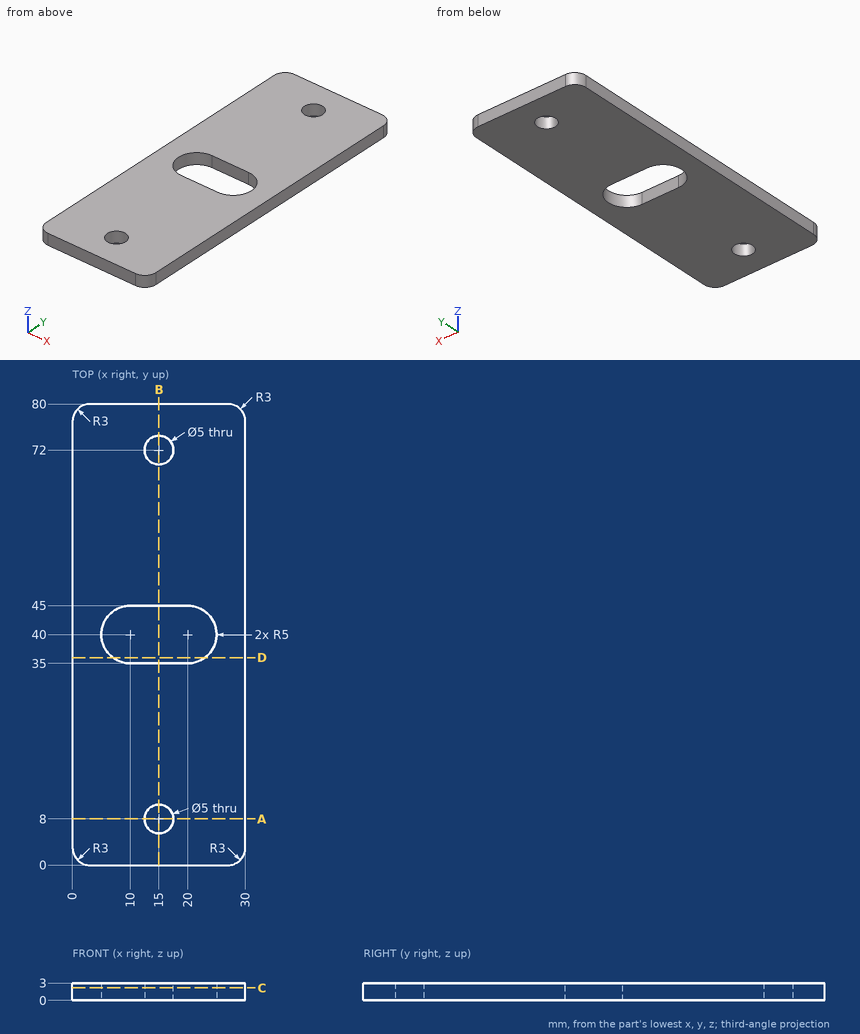
Could you check a few things on this drawing? It's one solid part, dimensions in mm from its lowest x, y, z. Coordinates: 2 decimals unless noted, no trailing zeros. Loops run counter-clockwise (first coordinate to the right, second up) from the corner with the lowest first, then second, coordinate; pieces in that order, holes last.
1. I need wall thicknesses on L1, parallel to Y at x = 15, z = 0.85; L2, parallel to X at y = 72, z = 2.15; L3, parallel to Y at x = 18, z = 2.2. Which ranges of each line are inside material? Lowest first, please.
2. Imagine slicing it at C-C (z = 2.15). Please give me the cut outline in (x, y).
3. Imagine slicing it at D-D (y = 36). Please give me the cut outline in (x, z), and give its area (3 significant figures).
4. Imagine slicing it at B-B (x = 15). Please give me the cut outline in (y, z).
5. Imagine slicing it at A-A (y = 8). Please give me the cut outline in (x, z).
Computed values:
1. L1: y = 0 to 5.5, 10.5 to 35, 45 to 69.5, 74.5 to 80
1. L2: x = 0 to 12.5, 17.5 to 30
1. L3: y = 0 to 35, 45 to 80
2. outline: (0, 3) arc R3 ccw to (3, 0) - (27, 0) arc R3 ccw to (30, 3) - (30, 77) arc R3 ccw to (27, 80) - (3, 80) arc R3 ccw to (0, 77) - close; hole (10, 35) - (20, 35) arc R5 ccw to (20, 45) - (10, 45) arc R5 ccw to start; hole circle Ø5 at (15, 8); hole circle Ø5 at (15, 72)
3. outline: (0, 0) - (7, 0) - (7, 3) - (0, 3) - close; (23, 0) - (30, 0) - (30, 3) - (23, 3) - close
3. area: 42.0 mm2
4. outline: (0, 0) - (5.5, 0) - (5.5, 3) - (0, 3) - close; (10.5, 0) - (35, 0) - (35, 3) - (10.5, 3) - close; (45, 0) - (69.5, 0) - (69.5, 3) - (45, 3) - close; (74.5, 0) - (80, 0) - (80, 3) - (74.5, 3) - close
5. outline: (0, 0) - (12.5, 0) - (12.5, 3) - (0, 3) - close; (17.5, 0) - (30, 0) - (30, 3) - (17.5, 3) - close
